```python
from build123d import *

# Parameters (mm, degrees)
F1_DEPTH = 10
F2_R     = 4.25
F3_DEPTH = 25


with BuildPart() as f1:
    # F0 (on Front) → F1 (new body, symmetric)
    with BuildSketch(Plane.XZ):
        Polygon((-60, 20), (-60, 0), (-35.6890111572, 0), (0, 89.222527893), (0, 120), (-20, 120), align=None)
    extrude(amount=F1_DEPTH, both=True)

    # F2 (on face) → F3 (cut)
    with BuildSketch(Plane(origin=(0, 0, 0), x_dir=(1, 0, 0), z_dir=(0, 0, -1))):
        with Locations((-49, 0)):
            Circle(F2_R)
    extrude(amount=-F3_DEPTH, mode=Mode.SUBTRACT)


solid = f1.part
```
Model file for the job. Use its own axes, mm. A direction names the side the tool comes from. Coordinates: 2 decimals unless noted, no trailing zeros. Loops run counter-clockwise (first coordinate to the right, second up) from the corner with the lowest first, then second, coordinate; pieces in that order, holes last. Notation, with made-up numbers: (-16.75, 1) - (6.25, 1) arc R27 cw to (6.25, 22) - close; hole circle Ø4 at (44.25, -8.5). An arc over 180 degrees is marked (long way). Write item = value, one per line. Start each with the question number.
Item 1: Saw through at B-B, the plane y = 0. List the corners of the cut face in (x, z), then the cut area to 3 significant figures.
Item 2: Pull direction Y, two halves, no side cores. Call faces 3 (the face through (-30, -10, 61)), 4 (the face through (-49, 0, 25)), 5 (the face through (-10, 0, 120)): +Y half, -Y half, draft (parallel to the pull), parting line (faces both ways), or undercut.
Item 3: Saw through at A-A, the plane x = -47. List the corners of the cut face in (y, z), then the cut area to 4 significant figures.
Item 4: Saw through at C-C, the plane z = 105.5. List the corners of the cut face in (x, y), then the cut area to 3 significant figures.
Item 5: Drop flat-ended pins along their axis: pin 1 Ø3 at (y, z) = (-2.5, 61) entering from -X; pin 2 Ø2 at (x, z) = (-17.5, 41.5) entering from +Y. Give the stop position or say it passes through.
Item 6: Saw through at D-D, the plane z = 17.5. List the corners of the cut face in (x, y).
Item 7: 3-axis set-ups, long thin cutter, end or side, ignore diameter. For faces 1 (the face through (0, 0, 104)), 2 (the face through (-53.246, -0.187, 12.325)): which of +Z, -Z, +X, -X, +Y, -Y reach the whole face in a straight line?
Item 8: Wall check: probe 1 along Y at (x, z) = (-49, 9.25); probe 2 along X at (y, z) = (0, 10.5); probe 3 along X at (y, z) = (0, 7.5). Give the ranges that are in metal, low to high. Write a range as [from, to].
Answers:
q1.outline = (-60, 0) - (-53.25, 0) - (-53.25, 25) - (-44.75, 25) - (-44.75, 0) - (-35.69, 0) - (0, 89.22) - (0, 120) - (-20, 120) - (-60, 20) - close
q1.area = 3,400 mm2
q2.face_3 = -Y half
q2.face_4 = undercut
q2.face_5 = draft
q3.outline = (-10, 0) - (-3.75, 0) - (-3.75, 25) - (3.75, 25) - (3.75, 0) - (10, 0) - (10, 52.5) - (-10, 52.5) - close
q3.area = 862.5 mm2
q4.outline = (-25.8, -10) - (0, -10) - (0, 10) - (-25.8, 10) - close
q4.area = 516 mm2
q5.pin_1 = -44.2
q5.pin_2 = through
q6.outline = (-60, -10) - (-28.69, -10) - (-28.69, 10) - (-60, 10) - close; hole circle Ø8.5 at (-49, 0)
q7.face_1 = +Z, -Z, +X, +Y, -Y
q7.face_2 = -Z
q8.probe_1 = [-10, -4.25], [4.25, 10]
q8.probe_2 = [-60, -53.25], [-44.75, -31.49]
q8.probe_3 = [-60, -53.25], [-44.75, -32.69]
